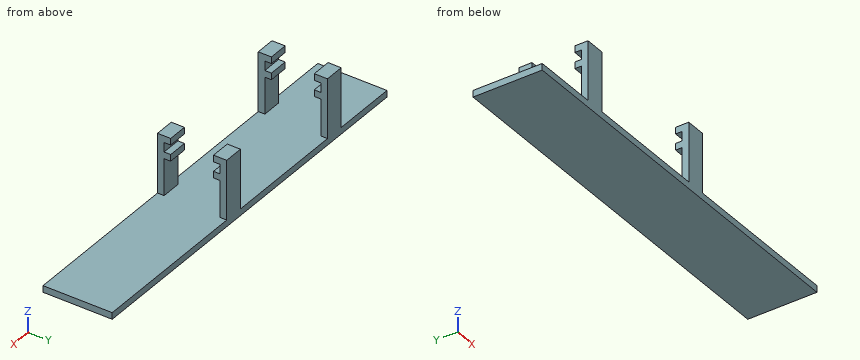
```python
from build123d import *

# Parameters (mm, degrees)
SKETCH1_W           = 60
SKETCH1_H           = 10.5
BOSS_EXTRUDE1_DEPTH = 1
SKETCH2_W           = 3
SKETCH2_H           = 10
BOSS_EXTRUDE2_DEPTH = 1
SKETCH3_W           = 3
SKETCH3_H           = 3.43
BOSS_EXTRUDE3_DEPTH = 1
SKETCH4_W           = 3
SKETCH4_H           = 1.43
CUT_EXTRUDE1_DEPTH  = 1
SKETCH6_W           = 3
SKETCH6_H           = 10
BOSS_EXTRUDE4_DEPTH = 1
SKETCH7_W           = 3
SKETCH7_H           = 3.43
BOSS_EXTRUDE5_DEPTH = 1
SKETCH8_W           = 3
SKETCH8_H           = 1.43
CUT_EXTRUDE2_DEPTH  = 1
SKETCH9_W           = 3
SKETCH9_H           = 10
BOSS_EXTRUDE6_DEPTH = 1
SKETCH10_W          = 3
SKETCH10_H          = 3.43
BOSS_EXTRUDE7_DEPTH = 1
SKETCH11_W          = 3
SKETCH11_H          = 1.43
CUT_EXTRUDE3_DEPTH  = 1
SKETCH12_W          = 3
SKETCH12_H          = 10
BOSS_EXTRUDE8_DEPTH = 1
SKETCH13_W          = 3
SKETCH13_H          = 3.43
BOSS_EXTRUDE9_DEPTH = 1
SKETCH14_W          = 3
SKETCH14_H          = 1.43
CUT_EXTRUDE4_DEPTH  = 1


with BuildPart() as part:
    # Sketch1 → Boss-Extrude1 (new body)
    with BuildSketch(Plane.XY):
        with Locations((30, 5.25)):
            Rectangle(SKETCH1_W, SKETCH1_H)
    extrude(amount=BOSS_EXTRUDE1_DEPTH)

    # Sketch2 → Boss-Extrude2 (add)
    with BuildSketch(Plane.XZ):
        with Locations((11.5, 5)):
            Rectangle(SKETCH2_W, SKETCH2_H)
    extrude(amount=-BOSS_EXTRUDE2_DEPTH)

    # Sketch3 → Boss-Extrude3 (add)
    with BuildSketch(Plane(origin=(0, 1, 0), x_dir=(1, 0, 0), z_dir=(0, 1, 0))):
        with Locations((11.5, -8.285)):
            Rectangle(SKETCH3_W, SKETCH3_H)
    extrude(amount=BOSS_EXTRUDE3_DEPTH)

    # Sketch4 → Cut-Extrude1 (cut)
    with BuildSketch(Plane(origin=(0, 2, 0), x_dir=(1, 0, 0), z_dir=(0, 1, 0))):
        with Locations((11.5, -8.285)):
            Rectangle(SKETCH4_W, SKETCH4_H)
    extrude(amount=-CUT_EXTRUDE1_DEPTH, mode=Mode.SUBTRACT)

    # Sketch6 → Boss-Extrude4 (add)
    with BuildSketch(Plane(origin=(0, 10.5, 0), x_dir=(1, 0, 0), z_dir=(0, 1, 0))):
        with Locations((11.5, -5)):
            Rectangle(SKETCH6_W, SKETCH6_H)
    extrude(amount=-BOSS_EXTRUDE4_DEPTH)

    # Sketch7 → Boss-Extrude5 (add)
    with BuildSketch(Plane.XZ.offset(-9.5)):
        with Locations((11.5, 8.285)):
            Rectangle(SKETCH7_W, SKETCH7_H)
    extrude(amount=BOSS_EXTRUDE5_DEPTH)

    # Sketch8 → Cut-Extrude2 (cut)
    with BuildSketch(Plane.XZ.offset(-8.5)):
        with Locations((11.5, 8.285)):
            Rectangle(SKETCH8_W, SKETCH8_H)
    extrude(amount=-CUT_EXTRUDE2_DEPTH, mode=Mode.SUBTRACT)

    # Sketch9 → Boss-Extrude6 (add)
    with BuildSketch(Plane.XZ):
        with Locations((33.5, 5)):
            Rectangle(SKETCH9_W, SKETCH9_H)
    extrude(amount=-BOSS_EXTRUDE6_DEPTH)

    # Sketch10 → Boss-Extrude7 (add)
    with BuildSketch(Plane(origin=(0, 1, 0), x_dir=(1, 0, 0), z_dir=(0, 1, 0))):
        with Locations((33.5, -8.285)):
            Rectangle(SKETCH10_W, SKETCH10_H)
    extrude(amount=BOSS_EXTRUDE7_DEPTH)

    # Sketch11 → Cut-Extrude3 (cut)
    with BuildSketch(Plane(origin=(0, 2, 0), x_dir=(1, 0, 0), z_dir=(0, 1, 0))):
        with Locations((33.5, -8.285)):
            Rectangle(SKETCH11_W, SKETCH11_H)
    extrude(amount=-CUT_EXTRUDE3_DEPTH, mode=Mode.SUBTRACT)

    # Sketch12 → Boss-Extrude8 (add)
    with BuildSketch(Plane(origin=(0, 10.5, 0), x_dir=(1, 0, 0), z_dir=(0, 1, 0))):
        with Locations((33.5, -5)):
            Rectangle(SKETCH12_W, SKETCH12_H)
    extrude(amount=-BOSS_EXTRUDE8_DEPTH)

    # Sketch13 → Boss-Extrude9 (add)
    with BuildSketch(Plane.XZ.offset(-9.5)):
        with Locations((33.5, 8.285)):
            Rectangle(SKETCH13_W, SKETCH13_H)
    extrude(amount=BOSS_EXTRUDE9_DEPTH)

    # Sketch14 → Cut-Extrude4 (cut)
    with BuildSketch(Plane.XZ.offset(-8.5)):
        with Locations((33.5, 8.285)):
            Rectangle(SKETCH14_W, SKETCH14_H)
    extrude(amount=-CUT_EXTRUDE4_DEPTH, mode=Mode.SUBTRACT)


solid = part.part
```
For this review, take the finished solid that the model builds, in its own axes (mm). Round coordinates to 2 decimals unless told otherwise and drop trailing zeros. Write each loop counter-clockwise with the first axis right and the second up, starting at its lowest first coordinate (ties: lowest second). Pieces come first, ordered by that corner, then holes. Notation, with made-up numbers: M -26.75,35.25 L -15.75,35.25 A26 ccw -15.75,66.25 Z; hole C 61.5,58 d3. An arc over 180 degrees is marked long. One line per item, written item: value. Start each with the question number.
(1) Insertion check: pin 1 (2 mm diameter, centred on x = 11.5, y = 5.5, fed in from +Z); pin 2 (0.6 mm diameter, centred on y = 9.5, z = 6, fed in from -X); pin 3 (4 mm diameter, centred on y = 9.5, z = 7, fed in from +X). Each pin has a flat end and moves straight along its axis. Give the tip position at first contact, or say it passes through.
(2) We need section A-A (z = 3). Give the boundary of the cut face in (x, y).
(3) We need section C-C (x = 12). Give the boundary of the cut face in (y, z), and give its area (3 significant figures).
(4) Wall thickness on line 1 (Y direction, x = 12, z = 1.5); line 2 (Z direction, x = 41.5, y = 2.5); line 3 (X direction, y = 9, z = 7.5): over which ranges is each line inside the solid? List them lowest first.
(5) We need section D-D (y = 4.75). Give the boundary of the cut face in (x, z), and give its area (3 significant figures).
(6) We need section B-B (y = 9). Give the boundary of the cut face in (x, z).
Result:
1. pin 1: z = 1
1. pin 2: x = 10
1. pin 3: x = 35
2. outline: M 10,0 L 13,0 L 13,1 L 10,1 Z; M 10,9.5 L 13,9.5 L 13,10.5 L 10,10.5 Z; M 32,0 L 35,0 L 35,1 L 32,1 Z; M 32,9.5 L 35,9.5 L 35,10.5 L 32,10.5 Z
3. outline: M 0,0 L 10.5,0 L 10.5,10 L 8.5,10 L 8.5,9 L 9.5,9 L 9.5,7.57 L 8.5,7.57 L 8.5,6.57 L 9.5,6.57 L 9.5,1 L 1,1 L 1,6.57 L 2,6.57 L 2,7.57 L 1,7.57 L 1,9 L 2,9 L 2,10 L 0,10 Z
3. area: 32.5 mm²
4. line 1: 0 to 1, 9.5 to 10.5
4. line 2: 0 to 1
4. line 3: 10 to 13, 32 to 35
5. outline: M 0,0 L 60,0 L 60,1 L 0,1 Z
5. area: 60.0 mm²
6. outline: M 0,0 L 60,0 L 60,1 L 0,1 Z; M 10,6.57 L 13,6.57 L 13,7.57 L 10,7.57 Z; M 10,9 L 13,9 L 13,10 L 10,10 Z; M 32,6.57 L 35,6.57 L 35,7.57 L 32,7.57 Z; M 32,9 L 35,9 L 35,10 L 32,10 Z
